from build123d import *

# Parameters (mm, degrees)
F0_R     = 38.1703800994
F1_DEPTH = 8.0033224076
F3_T     = -5.08
F4_DEPTH = 12.0424441993
F5_SIZE  = 5.08


# Not quite as in the source:
# - a fillet or chamfer that OpenCascade refuses, or shapes differently, is made with other operations: its cross-section is extruded or revolved along the edge and cut away or added


with BuildPart() as f1:
    # F0 (on Top) → F1 (new body)
    with BuildSketch(Plane.XY):
        Circle(F0_R)
    extrude(amount=F1_DEPTH)

    # F2: fillet of radius 13.1324976857 on 1 edges, made by hand

    # F2_s1 → F2_t2 (revolve, cut)
    with BuildSketch(Plane.XZ):
        with BuildLine():
            ThreePointArc((38.1703800994, 0), (33.3302233857, 5.821198641), (26.0809609061, 8.0033224076))
            Line((26.0809609061, 8.0033224076), (38.1703800994, 8.0033224076))
            Line((38.1703800994, 8.0033224076), (38.1703800994, 0))
        make_face()
    revolve(axis=Axis((0, 0, 8.0033224076), (0, 0, 1)), mode=Mode.SUBTRACT)

    # F3
    f3_openings = [f1.faces().sort_by_distance(p)[0] for p in [
        (0, 0, 0),
    ]]
    offset(amount=F3_T, openings=f3_openings)

    # F4 (add): a face of the model
    f4_faces = [f1.faces().sort_by_distance(p)[0] for p in [
        (0, 0, 8.0033224076),
    ]]
    extrude(f4_faces, amount=F4_DEPTH)

    # F5
    f5_edges = [f1.edges().sort_by_distance(p)[0] for p in [
        (-26.080961, 0, 20.045767),
    ]]
    chamfer(f5_edges, length=F5_SIZE)


solid = f1.part
Design review of the part built by this model. Coordinates are the model's own, in mm. A direction names the side the tool comes from. Round coordinates to 2 decimals unless told otherwise and drop trailing zeros. Loops run counter-clockwise (first coordinate to the right, second up) from the corner with the lowest first, then second, coordinate; pieces in that order, holes last. Notation, with made-up numbers: M 47,62 L 92,62 A23 cw 92,81 Z; hole C 2,-40 d5. An arc over 180 degrees is marked long. Answer as a JSON object with one key per item and string values.
Item 1: Wall thickness on L1, parallel to Z at x = 9, y = -11.5; L2, parallel to Z at x = 20.5, y = 16.5; L3, parallel to Y at x = -23.5, z = 1.5: over which ranges is each line inside the solid? List them lowest first. Write a range as from..to.
Answer sheet:
{"L1": "z = 2.92..20.05", "L2": "z = 2.92..8", "L3": "y = -29.12..-19.68, 19.68..29.12"}
Item 2: We need section D-D on z = 2. Give the boundary of the cut face in (x, y).
Answer sheet:
{"outline": "C 0,0 d74.22; hole C 0,0 d59.65"}
Item 3: The part is to be moulded in two halves that separate along X. For faces 1 (the flat face through (0, 0, 2.923)), 2 (the flat face through (-31.3, 8.7, 0)), 3 (the conical face through (-16.86, -12.93, 19.8)), say which applies: pulls with the +X half, pulls with the -X half, needs draft (parallel to the pull), parting line crosses it, or undercut.
Answer sheet:
{"face 1": "undercut", "face 2": "needs draft", "face 3": "parting line crosses it"}
Item 4: Clearance check with flat-ended pins moving along their axes: P1, Ø1, axis at x = -3.5, z = 15, coming from the +Y side; P2, Ø6, axis at y = -17, z = 14, coming from the +X side; P3, Ø4, axis at x = -8, z = 10.5, coming from the +Y side. State where each tip first meets the part, or that it passes through.
Answer sheet:
{"P1": "stops at y = 25.91", "P2": "stops at x = 22", "P3": "stops at y = 25.38"}
Item 5: We need section C-C on z = 13. Give the boundary of the cut face in (x, y).
Answer sheet:
{"outline": "C 0,0 d52.16"}
Item 6: We need section A-A on x = 0. Give the boundary of the cut face in (y, z) (1 decimal).
Answer sheet:
{"outline": "M -38.2,0 L -32.3,0 A8.1 cw -26.1,2.9 L 26.1,2.9 A8.1 cw 32.3,0 L 38.2,0 A13.1 ccw 26.1,8 L 26.1,15 L 21,20 L -21,20 L -26.1,15 L -26.1,8 A13.1 ccw Z"}
Item 7: Machinability: for faces 4 (the flat face through (0, 0, 20.046)), 5 (the cylindrical face through (24.877, 7.834, 11.436)), which of the approach directions +Z, -Z, +X, -X, +Y, -Y give a long, thin tool a straight path to every point of the face, cutting with its end or side? Answer none if there is none.
Answer sheet:
{"face 4": "+Z, +X, -X, +Y, -Y", "face 5": "+Z"}
